from build123d import *

# Parameters (mm, degrees)
CASCA1_T                 = -0.9
RESSALTO_EXTRUS_O1_DEPTH = 9
FILETE1_R                = 1
ESBO_O3_R                = 2.38125
CORTE_EXTRUS_O1_DEPTH    = 39.143338529


with BuildPart() as part:
    # Esboço1 → Revolução1 (revolve)
    with BuildSketch(Plane.XY, mode=Mode.PRIVATE) as revolu_o1_sk:
        Polygon((0, 0), (13.5, 0), (8.5, 4), (14, 10), (7.5, 15), (7.5, 24), (0, 24), align=None)
    revolve(revolu_o1_sk.sketch.rotate(Axis((0, 24, 0), (0, -1, 0)), 180), axis=Axis((0, 24, 0), (0, -1, 0)))

    # Casca1
    casca1_openings = [part.faces().sort_by_distance(p)[0] for p in [
        (0, 0, 0),
    ]]
    offset(amount=CASCA1_T, openings=casca1_openings, kind=Kind.INTERSECTION)

    # Esboço2 → Ressalto-extrusão1 (add)
    with BuildSketch(Plane(origin=(0, 24, 0), x_dir=(1, 0, 0), z_dir=(0, 1, 0))):
        Polygon((2.496763598, 3.885808136), (-2.11682676, 4.105164771), (-4.613590359, 0.219356636), (-2.496763598, -3.885808136), (2.11682676, -4.105164771), (4.613590359, -0.219356636), align=None)
    extrude(amount=RESSALTO_EXTRUS_O1_DEPTH)

    # Filete1
    filete1_edges = [part.edges().sort_by_distance(p)[0] for p in [
        (7.5, 15, 0),
        (14, 10, 0),
        (8.5, 4, 0),
    ]]
    fillet(filete1_edges, radius=FILETE1_R)

    # Esboço3 → Corte-extrusão1 (cut, through all)
    with BuildSketch(Plane(origin=(0, 33, 0), x_dir=(1, 0, 0), z_dir=(0, 1, 0))):
        with Locations(Location((0, 0, 0), (0, 0, 270))):
            Circle(ESBO_O3_R)
    extrude(amount=-CORTE_EXTRUS_O1_DEPTH, mode=Mode.SUBTRACT)


solid = part.part
The listing builds one solid part. Answer for the finished solid, in the listing's coordinates (mm). A direction names the side the tool comes from. Round coordinates to 2 decimals unless told otherwise and drop trailing zeros. Write each loop counter-clockwise with the first axis right and the second up, starting at its lowest first coordinate (ties: lowest second). Pieces come first, ordered by that corner, then holes. Notation, with made-up numbers: M -27,78 L -16,78 A9 ccw -16,92 Z; hole C 6,74.25 d3. An arc over 180 degrees is marked long. Write each question's results on one line, items separated by ' | '. Start each with the question number.
Item 1: A cutting plane is placed at A-A on y = 28.5. Write down the section's boundary in (x, z), and give its area (3 significant figures).
Item 2: For a pull along Z with two mould halves and no side action, classify faces 5 (the face through (-3.57, 28.437, 1.804)), 6 (the face through (0.222, 28.437, -3.994)), 7 (the face through (4.864, 18.888, -4.461)), 8 (the face through (-3.425, 3.709, 6.585)) as pulls with the +Z half, pulls with the -Z half, needs draft (parallel to the pull), parting line crosses it, or undercut.
Item 3: For faces 1 (the face through (-3, 23.1, 0)), 2 (the face through (-9.1, 3.17, -2.86)), 3 (the face through (-0.222, 28.437, 3.994)), 4 (the face through (-3.2, 24, 3.2)), determine the directions among +Z, -Z, +X, -X, +Y, -Y from which every point of the face is accessible in a straight line to the end or side of a thin tool.
Item 4: A cutting plane is placed at C-C on y = 11.5. Write down the section's boundary in (x, z).
Item 5: Straight lines are drawn through the part: L1, parallel to Y at x = -6.5, z = -7.25; L2, parallel to Y at x = -6.25, z = 7.25; L3, parallel to Z at x = 0, y = 17. For each, find the intervals that lie inside material, in ascending order. Write a range as [from, to].
Item 6: A cutting plane is placed at B-B on y = 22.5. Write down the section's boundary in (x, z).
Item 7: Flat-ended cylindrical pins translate along their axes: pin 1 Ø10 at (y, z) = (4.5, 10) entering from +X; pin 2 Ø6 at (x, z) = (0, 0) entering from +Y; pin 3 Ø14.5 at (x, z) = (1.5, -0.5) entering from -Y; pin 4 Ø8 at (x, z) = (-5, -2.5) entering from -Y. Find the tip coordinate at first contact, or state that the pin passes through.
Check sheet entries:
1) outline: M -4.61,-0.22 L -2.12,-4.11 L 2.5,-3.89 L 4.61,0.22 L 2.12,4.11 L -2.5,3.89 Z; hole C 0,0 d4.76 | area: 37.6 mm²
2) face 5: pulls with the +Z half | face 6: pulls with the -Z half | face 7: undercut | face 8: undercut
3) face 1: -Y | face 2: none | face 3: +Z, -X, +Y | face 4: +Y
4) outline: C 0,0 d24.1; hole C 0,0 d21.15
5) L1: [1.86, 3.01], [5.35, 6.68], [12.14, 13.28] | L2: [1.99, 3.14], [5.17, 6.5], [12.27, 13.41] | L3: [-7.5, -6.6], [6.6, 7.5]
6) outline: C 0,0 d15; hole C 0,0 d13.2
7) pin 1: x = 11 | pin 2: y = 33 | pin 3: y = 2.58 | pin 4: y = 1.98
